Here's how the part is built. I have some questions about the finished solid (model axes, mm). Coordinates: 2 decimals unless noted, no trailing zeros.
(1) For pin 1 Ø3 at (x, y) = (3, -6) entering from +Z; pin 2 Ø0.8 at (y, z) = (-18.5, -217.5) entering from -X; pin 3 Ø2 at (x, y) = (-7, -20.5) entering from +Z; pin 4 Ø1.4 at (x, z) = (1, -107.5) entering from -Y, each with a flat end and sliding along its axis, tell me the tip position at first contact or that it passes through.
(2) Imagine slicing it at A-A, the plane z = -76.5. State how many separate pieces and enclosed holes the cut face has, plus the area to 3 significant figures.
(3) Please list where these lines run through material, in increasing order: probe 1 along Y at (x, z) = (0, -164); probe 2 along Y at (x, z) = (0.5, -260); probe 3 along Y at (x, z) = (8.25, -264).
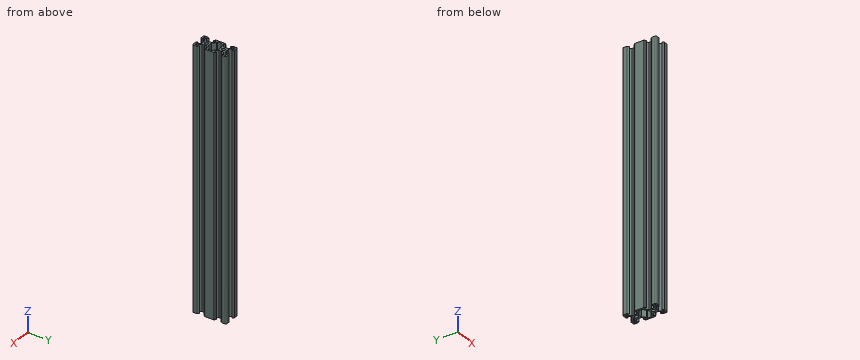
```python
from build123d import *

# Parameters (mm, degrees)
SKETCH2_R           = 2.1
BOSS_EXTRUDE1_DEPTH = 310


with BuildPart() as part:
    # Sketch2 → Boss-Extrude1 (new body)
    with BuildSketch(Plane.XY):
        with BuildLine():
            Line((-0.1, 3.9), (0, 3.8))
            Line((0, 3.8), (0.1, 3.9))
            Line((0.1, 3.9), (2.840365134, 3.9))
            Line((2.840365134, 3.9), (5.5, 6.558825842))
            Line((5.5, 6.558825842), (5.5, 8.197505675))
            Line((5.5, 8.197505675), (2.89, 8.197505675))
            Line((2.89, 8.197505675), (2.89, 8.307505675))
            Line((2.89, 8.307505675), (4.348614357, 9.766120032))
            ThreePointArc((4.348614357, 9.766120032), (4.604908803, 9.937370505), (4.907228714, 9.997505675))
            Line((4.907228714, 9.997505675), (8.5, 9.997505675))
            ThreePointArc((8.5, 9.997505675), (9.560660172, 9.558165846), (10, 8.497505675))
            Line((10, 8.497505675), (10, 4.904734389))
            ThreePointArc((10, 4.904734389), (9.939864831, 4.602414477), (9.768614357, 4.346120032))
            Line((9.768614357, 4.346120032), (8.31, 2.887505675))
            Line((8.31, 2.887505675), (8.2, 2.887505675))
            Line((8.2, 2.887505675), (8.2, 5.497505675))
            Line((8.2, 5.497505675), (6.56, 5.497505675))
            Line((6.56, 5.497505675), (3.9, 2.83831481))
            Line((3.9, 2.83831481), (3.9, 0.1))
            Line((3.9, 0.1), (3.8, 0))
            Line((3.8, 0), (3.9, -0.1))
            Line((3.9, -0.1), (3.9, -2.84))
            Line((3.9, -2.84), (6.56, -5.5))
            Line((6.56, -5.5), (8.2, -5.5))
            Line((8.2, -5.5), (8.2, -2.89))
            Line((8.2, -2.89), (8.31, -2.89))
            Line((8.31, -2.89), (9.765685425, -4.345685425))
            ThreePointArc((9.765685425, -4.345685425), (9.939103626, -4.605224104), (10, -4.91137085))
            Line((10, -4.91137085), (10, -15.08862915))
            ThreePointArc((10, -15.08862915), (9.939103626, -15.394775896), (9.765685425, -15.654314575))
            Line((9.765685425, -15.654314575), (8.31, -17.11))
            Line((8.31, -17.11), (8.2, -17.11))
            Line((8.2, -17.11), (8.2, -14.5))
            Line((8.2, -14.5), (6.56, -14.5))
            Line((6.56, -14.5), (3.9, -17.16))
            Line((3.9, -17.16), (3.9, -19.9))
            Line((3.9, -19.9), (3.8, -20))
            Line((3.8, -20), (3.9, -20.1))
            Line((3.9, -20.1), (3.9, -22.83831481))
            Line((3.9, -22.83831481), (6.56, -25.497505675))
            Line((6.56, -25.497505675), (8.2, -25.497505675))
            Line((8.2, -25.497505675), (8.2, -22.887505675))
            Line((8.2, -22.887505675), (8.31, -22.887505675))
            Line((8.31, -22.887505675), (9.768614357, -24.346120032))
            ThreePointArc((9.768614357, -24.346120032), (9.939864831, -24.602414477), (10, -24.904734389))
            Line((10, -24.904734389), (10, -28.497505675))
            ThreePointArc((10, -28.497505675), (9.560660172, -29.558165846), (8.5, -29.997505675))
            Line((8.5, -29.997505675), (4.907228714, -29.997505675))
            ThreePointArc((4.907228714, -29.997505675), (4.604908803, -29.937370505), (4.348614357, -29.766120032))
            Line((4.348614357, -29.766120032), (2.89, -28.307505675))
            Line((2.89, -28.307505675), (2.89, -28.197505675))
            Line((2.89, -28.197505675), (5.5, -28.197505675))
            Line((5.5, -28.197505675), (5.5, -26.558825842))
            Line((5.5, -26.558825842), (2.840365134, -23.9))
            Line((2.840365134, -23.9), (0.1, -23.9))
            Line((0.1, -23.9), (0, -23.8))
            Line((0, -23.8), (-0.1, -23.9))
            Line((-0.1, -23.9), (-2.840365134, -23.9))
            Line((-2.840365134, -23.9), (-5.5, -26.558825842))
            Line((-5.5, -26.558825842), (-5.5, -28.197505675))
            Line((-5.5, -28.197505675), (-2.89, -28.197505675))
            Line((-2.89, -28.197505675), (-2.89, -28.307505675))
            Line((-2.89, -28.307505675), (-4.348614357, -29.766120032))
            ThreePointArc((-4.348614357, -29.766120032), (-4.604908803, -29.937370505), (-4.907228714, -29.997505675))
            Line((-4.907228714, -29.997505675), (-8.5, -29.997505675))
            ThreePointArc((-8.5, -29.997505675), (-9.560660172, -29.558165846), (-10, -28.497505675))
            Line((-10, -28.497505675), (-10, -24.904734389))
            ThreePointArc((-10, -24.904734389), (-9.939864831, -24.602414477), (-9.768614357, -24.346120032))
            Line((-9.768614357, -24.346120032), (-8.31, -22.887505675))
            Line((-8.31, -22.887505675), (-8.2, -22.887505675))
            Line((-8.2, -22.887505675), (-8.2, -25.497505675))
            Line((-8.2, -25.497505675), (-6.56, -25.497505675))
            Line((-6.56, -25.497505675), (-3.9, -22.83831481))
            Line((-3.9, -22.83831481), (-3.9, -20.1))
            Line((-3.9, -20.1), (-3.8, -20))
            Line((-3.8, -20), (-3.9, -19.9))
            Line((-3.9, -19.9), (-3.9, -17.16))
            Line((-3.9, -17.16), (-6.56, -14.5))
            Line((-6.56, -14.5), (-8.2, -14.5))
            Line((-8.2, -14.5), (-8.2, -17.11))
            Line((-8.2, -17.11), (-8.31, -17.11))
            Line((-8.31, -17.11), (-9.765685425, -15.654314575))
            ThreePointArc((-9.765685425, -15.654314575), (-9.939103626, -15.394775896), (-10, -15.08862915))
            Line((-10, -15.08862915), (-10, -4.91137085))
            ThreePointArc((-10, -4.91137085), (-9.939103626, -4.605224104), (-9.765685425, -4.345685425))
            Line((-9.765685425, -4.345685425), (-8.31, -2.89))
            Line((-8.31, -2.89), (-8.2, -2.89))
            Line((-8.2, -2.89), (-8.2, -5.5))
            Line((-8.2, -5.5), (-6.56, -5.5))
            Line((-6.56, -5.5), (-3.9, -2.84))
            Line((-3.9, -2.84), (-3.9, -0.1))
            Line((-3.9, -0.1), (-3.8, 0))
            Line((-3.8, 0), (-3.9, 0.1))
            Line((-3.9, 0.1), (-3.9, 2.83831481))
            Line((-3.9, 2.83831481), (-6.56, 5.497505675))
            Line((-6.56, 5.497505675), (-8.2, 5.497505675))
            Line((-8.2, 5.497505675), (-8.2, 2.887505675))
            Line((-8.2, 2.887505675), (-8.31, 2.887505675))
            Line((-8.31, 2.887505675), (-9.768614357, 4.346120032))
            ThreePointArc((-9.768614357, 4.346120032), (-9.939864831, 4.602414477), (-10, 4.904734389))
            Line((-10, 4.904734389), (-10, 8.497505675))
            ThreePointArc((-10, 8.497505675), (-9.560660172, 9.558165846), (-8.5, 9.997505675))
            Line((-8.5, 9.997505675), (-4.907228714, 9.997505675))
            ThreePointArc((-4.907228714, 9.997505675), (-4.604908803, 9.937370505), (-4.348614357, 9.766120032))
            Line((-4.348614357, 9.766120032), (-2.89, 8.307505675))
            Line((-2.89, 8.307505675), (-2.89, 8.197505675))
            Line((-2.89, 8.197505675), (-5.5, 8.197505675))
            Line((-5.5, 8.197505675), (-5.5, 6.558825842))
            Line((-5.5, 6.558825842), (-2.840365134, 3.9))
            Line((-2.840365134, 3.9), (-0.1, 3.9))
        make_face()
        Circle(SKETCH2_R, mode=Mode.SUBTRACT)
        with Locations((0, -20)):
            Circle(SKETCH2_R, mode=Mode.SUBTRACT)
        Polygon((-7.66, 6.567505675), (-6.57, 7.657505675), (-6.57, 8.197505675), (-8.2, 8.197505675), (-8.2, 6.567505675), align=None, mode=Mode.SUBTRACT)
        Polygon((-0.1, -3.9), (0, -3.8), (0.1, -3.9), (2.840365134, -3.9), (6.24, -7.299634866), (8.2, -7.299634866), (8.2, -12.700365134), (6.24, -12.700365134), (2.840365134, -16.1), (0.1, -16.1), (0, -16.2), (-0.1, -16.1), (-2.840365134, -16.1), (-6.24, -12.700365134), (-8.2, -12.700365134), (-8.2, -7.299634866), (-6.24, -7.299634866), (-2.840365134, -3.9), align=None, mode=Mode.SUBTRACT)
        Polygon((8.2, 6.567505675), (7.66, 6.567505675), (6.57, 7.657505675), (6.57, 8.197505675), (8.2, 8.197505675), align=None, mode=Mode.SUBTRACT)
        Polygon((7.66, -26.567505675), (6.57, -27.657505675), (6.57, -28.197505675), (8.2, -28.197505675), (8.2, -26.567505675), align=None, mode=Mode.SUBTRACT)
        Polygon((-8.2, -26.567505675), (-7.66, -26.567505675), (-6.57, -27.657505675), (-6.57, -28.197505675), (-8.2, -28.197505675), align=None, mode=Mode.SUBTRACT)
    extrude(amount=-BOSS_EXTRUDE1_DEPTH)


solid = part.part
```
Recorded:
1. pin 1: stops at z = 0
1. pin 2: stops at x = -3.9
1. pin 3: passes through
1. pin 4: stops at y = -23.9
2. separate pieces: 1
2. enclosed holes: 7
2. area: 291 mm2
3. probe 1: y = -23.8 to -22.1, -17.9 to -16.2, -3.8 to -2.1, 2.1 to 3.8
3. probe 2: y = -23.9 to -22.04, -17.96 to -16.1, -3.9 to -2.04, 2.04 to 3.9
3. probe 3: y = -30 to -22.89, -17.11 to -2.89, 2.89 to 10
